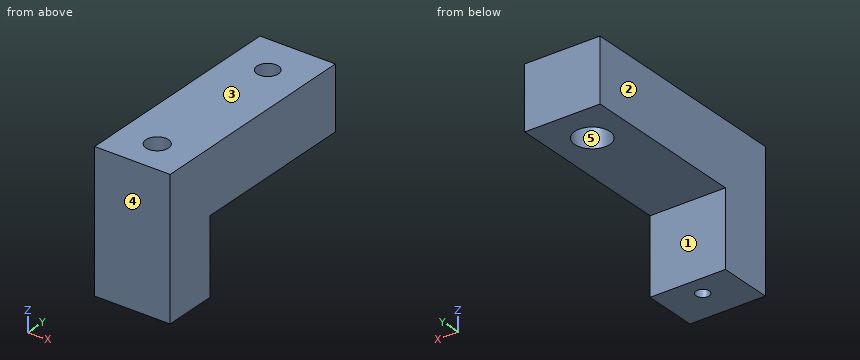
from build123d import *

# Parameters (mm, degrees)
EXTRUDE_1_DEPTH     = 30
SKETCH_2_R          = 2.65
CUT_EXTRUDE_1_DEPTH = 56
SKETCH_4_R          = 4.5
CUT_EXTRUDE_3_DEPTH = 42
SKETCH_5_R          = 4.25
CUT_EXTRUDE_4_DEPTH = 26
SKETCH_6_R          = 7
CUT_EXTRUDE_5_DEPTH = 8


with BuildPart() as part:
    # 草图1 → 凸台-拉伸1 (new body)
    with BuildSketch(Plane(origin=(0, 0, 0), x_dir=(0, 0, -1), z_dir=(1, 0, 0))):
        Polygon((-18.5, 8), (-18.5, -13.3), (-73.5, -13.3), (-73.5, 8), (-73.5, 75), (-48.5, 75), (-48.5, 8), align=None)
    extrude(amount=EXTRUDE_1_DEPTH)

    # 草图2 → 切除-拉伸1 (cut, through all)
    with BuildSketch(Plane(origin=(0, 0, 18.5), x_dir=(-1, 0, 0), z_dir=(0, 0, -1))):
        with Locations((-15, 0)):
            Circle(SKETCH_2_R)
    extrude(amount=-CUT_EXTRUDE_1_DEPTH, mode=Mode.SUBTRACT)

    # 草图4 → 切除-拉伸3 (cut, through all)
    with BuildSketch(Plane(origin=(0, 0, 32.5), x_dir=(-1, 0, 0), z_dir=(0, 0, -1))):
        with Locations((-15, 0)):
            Circle(SKETCH_4_R)
    extrude(amount=-CUT_EXTRUDE_3_DEPTH, mode=Mode.SUBTRACT)

    # 草图5 → 切除-拉伸4 (cut, through all)
    with BuildSketch(Plane(origin=(0, 0, 48.5), x_dir=(-1, 0, 0), z_dir=(0, 0, -1))):
        with Locations((-15, 59.038200963)):
            Circle(SKETCH_5_R)
    extrude(amount=-CUT_EXTRUDE_4_DEPTH, mode=Mode.SUBTRACT)

    # 草图6 → 切除-拉伸5 (cut)
    with BuildSketch(Plane(origin=(0, 0, 48.5), x_dir=(-1, 0, 0), z_dir=(0, 0, -1))):
        with Locations((-15, 59.038200963)):
            Circle(SKETCH_6_R)
    extrude(amount=-CUT_EXTRUDE_5_DEPTH, mode=Mode.SUBTRACT)


solid = part.part
Here's how the part is built. I have some questions about the finished solid (model axes, mm). Face numbers are marked on the shaded views. A direction names the side the tool comes from. Round coordinates to 2 decimals unless told otherwise and drop trailing zeros. Loops run counter-clockwise (first coordinate to the right, second up) from the corner with the lowest first, then second, coordinate; pieces in that order, holes last.
1. Which directions (+Z, -Z, +X, -X, +Y, -Y) give clear straight access to the entire face, cutting with the end or side of a thin tool? Please do the marked faces 1 and 2.
Answer list:
face 1: -Z, +X, -X, +Y
face 2: +Z, -Z, -X, +Y, -Y
2. If we section it at C-C on x = 15: Write out the boundary of the cut face in (y, z), plus the area to 3 significant figures.
Answer list:
outline: (-13.3, 18.5) - (-2.65, 18.5) - (-2.65, 32.5) - (-4.5, 32.5) - (-4.5, 73.5) - (-13.3, 73.5) - close; (2.65, 18.5) - (8, 18.5) - (8, 48.5) - (52.04, 48.5) - (52.04, 56.5) - (54.79, 56.5) - (54.79, 73.5) - (4.5, 73.5) - (4.5, 32.5) - (2.65, 32.5) - close; (63.29, 56.5) - (66.04, 56.5) - (66.04, 48.5) - (75, 48.5) - (75, 73.5) - (63.29, 73.5) - close
area: 2,150 mm2
3. If I drill on line 1 along Y through (x, z) = (15, 64); line 2 along Y through (x, z) = (15, 44.5); line 3 along Y through (x, z) = (15, 52.25), over which ranges is the centre line in solid material (lowest first)?
Answer list:
line 1: y = -13.3 to -4.5, 4.5 to 54.79, 63.29 to 75
line 2: y = -13.3 to -4.5, 4.5 to 8
line 3: y = -13.3 to -4.5, 4.5 to 52.04, 66.04 to 75
4. For P1, Ø15.5, axis at x = 12, y = 56, coming from the -Z side; P2, Ø15, axis at x = 12, z = 31.5, coming from the +Y side; P3, Ø5.5, axis at x = 15, y = 0, coming from the +Z side, each with a flat end and sliding along its axis, tell me the tip position at first contact or that it passes through.
Answer list:
P1: stops at z = 48.5
P2: stops at y = 8
P3: stops at z = 32.5
5. We'd pull the mould along Y, two halves only. Please class the marked faces 3, 4 and 5: +Y half, -Y half, draft (parallel to the pull), parting line (faces both ways), or undercut.
Answer list:
face 3: draft
face 4: -Y half
face 5: undercut
6. If we section it at A-A on y = 0: Write out the boundary of the cut face in (x, z).
Answer list:
outline: (0, 18.5) - (12.35, 18.5) - (12.35, 32.5) - (10.5, 32.5) - (10.5, 73.5) - (0, 73.5) - close; (17.65, 18.5) - (30, 18.5) - (30, 73.5) - (19.5, 73.5) - (19.5, 32.5) - (17.65, 32.5) - close
7. If we section it at D-D on x = 27: Write out the boundary of the cut face in (y, z).
Answer list:
outline: (-13.3, 18.5) - (8, 18.5) - (8, 48.5) - (75, 48.5) - (75, 73.5) - (-13.3, 73.5) - close
8. If we section it at B-B on z = 23.5: Write out the boundary of the cut face in (x, y), plus the area to 3 significant figures.
Answer list:
outline: (0, -13.3) - (30, -13.3) - (30, 8) - (0, 8) - close; hole circle Ø5.3 at (15, 0)
area: 617 mm2
